CAD build for the part. Positions are in the model's coordinates, mm. Round coordinates to 2 decimals unless told otherwise and drop trailing zeros. Loops run counter-clockwise (first coordinate to the right, second up) from the corner with the lowest first, then second, coordinate; pieces in that order, holes last. Notation, with made-up numbers: M -7,17 L 25,17 A25 cw 25,49 Z; hole C 3.25,11.25 d5. An arc over 180 degrees is marked long. Use a Markdown table: item, result. Add a question column.
(1) Wall check: L1, parallel to Y at x = 3.75, z = 0.3; L2, parallel to Y at x = -0.75, z = 4.7; L3, parallel to Y at x = 3.5, z = 0.95. Give the ranges that are in metal, low to high.
(2) Band-saw the part on D-D, the plane z = 2.75. Write the cut outline in (x, y), and give its area (3 significant figures).
(3) Band-saw the part on B-B, the plane y = -3. Write the cut outline in (x, z), and give its area (3 significant figures).
(4) Band-saw the part on C-C, the plane z = 3.65. Write the cut outline in (x, y).
(5) Band-saw the part on A-A, the plane x = 0. Write the cut outline in (y, z).
(6) Flat gauge pins, fed straight in: P1, Ø3, axis at y = 1, z = 1.5, coming from the -X side; P2, Ø1.5, axis at x = 1.5, z = 3.5, coming from the +Y side. Where does each tip first touch, or does it go through?
from build123d import *

# Parameters (mm, degrees)
SKETCH1_W                 = 34.29304938
SKETCH1_H                 = 54.588935748
BOSS_EXTRUDE1_DEPTH       = 2
SKETCH3_W                 = 33.162023886
SKETCH3_H                 = 45.144780362
BOSS_EXTRUDE3_DEPTH       = 19
BOSS_EXTRUDE3_TAPER       = 15
F_1_64_TAPPED_HOLE1_D     = 1.5113
F_1_64_TAPPED_HOLE1_DEPTH = 4.89712
F_1_64_TAPPED_HOLE1_TIP   = 0.454040327
SCALE2_SCALE              = 0.5
SCALE5_SCALE              = 0.5


with BuildPart() as part:
    # Sketch1 → Boss-Extrude1 (new body)
    with BuildSketch(Plane.XY):
        Rectangle(SKETCH1_W, SKETCH1_H)
    extrude(amount=BOSS_EXTRUDE1_DEPTH)

    # Sketch3 → Boss-Extrude3 (add)
    with BuildSketch(Plane.XY.offset(2)):
        Rectangle(SKETCH3_W, SKETCH3_H)
    extrude(amount=BOSS_EXTRUDE3_DEPTH, taper=BOSS_EXTRUDE3_TAPER)

    # #1-64 Tapped Hole1
    with Locations(Plane(origin=(15.000680777, 25.209477417, 2), x_dir=(1, 0, 0), z_dir=(0, 0, 1))):
        with Locations((0, 0), (-30.140256747, -0.069447596), (-30.487494728, -50.905088008), (-0.069447596, -50.835640411)):
            Hole(F_1_64_TAPPED_HOLE1_D / 2, depth=F_1_64_TAPPED_HOLE1_DEPTH)
            with Locations((0, 0, -(F_1_64_TAPPED_HOLE1_DEPTH + F_1_64_TAPPED_HOLE1_TIP / 2))):  # 118° drill point
                Cone(0, F_1_64_TAPPED_HOLE1_D / 2, F_1_64_TAPPED_HOLE1_TIP, mode=Mode.SUBTRACT)


with BuildPart() as part_1:
    # Scale2: scaled about (0, 0, 0)
    add(part.part.scale(SCALE2_SCALE))


with BuildPart() as part_2:
    # Scale5: scaled about (0, 0, 0)
    add(part_1.part.scale(SCALE5_SCALE))


solid = part_2.part
Return value:
| question | item | result |
|---|---|---|
| 1 | L1 | -6.82 to -6.59, -6.22 to 6.11, 6.49 to 6.82 |
| 1 | L2 | -4.52 to 4.52 |
| 1 | L3 | -5.52 to 5.52 |
| 2 | outline | M -3.54,-5.04 L 3.54,-5.04 L 3.54,5.04 L -3.54,5.04 Z |
| 2 | area | 71.4 mm^2 |
| 3 | outline | M -4.29,0 L 4.29,0 L 4.29,0.5 L 4.15,0.5 L 2.87,5.25 L -2.87,5.25 L -4.15,0.5 L -4.29,0.5 Z |
| 3 | area | 37.6 mm^2 |
| 4 | outline | M -3.3,-4.8 L 3.3,-4.8 L 3.3,4.8 L -3.3,4.8 Z |
| 5 | outline | M -6.82,0 L 6.82,0 L 6.82,0.5 L 5.64,0.5 L 4.37,5.25 L -4.37,5.25 L -5.64,0.5 L -6.82,0.5 Z |
| 6 | P1 | x = -4.29 |
| 6 | P2 | y = 5.04 |
